from build123d import *

# Parameters (mm, degrees)
SKETCH_1_W          = 117.5
SKETCH_1_H          = 26
EXTRUDE_1_DEPTH     = 1.6
SKETCH_2_R          = 2.2
EXTRUDE_4_DEPTH     = 6.9
SKETCH_3_R          = 1.5
CUT_EXTRUDE_2_DEPTH = 1.6
CUT_EXTRUDE_3_DEPTH = 1.6
SKETCH_5_W          = 20
SKETCH_5_H          = 9
EXTRUDE_5_DEPTH     = 9
SKETCH_6_W          = 18
SKETCH_6_H          = 7
CUT_EXTRUDE_4_DEPTH = 9
FILLET_1_R          = 1.5
CUT_EXTRUDE_5_DEPTH = 1.6
FILLET_2_R          = 1.5


with BuildPart() as part:
    # 草图1 → 凸台-拉伸1 (new body)
    with BuildSketch(Plane.XY):
        Rectangle(SKETCH_1_W, SKETCH_1_H)
    extrude(amount=EXTRUDE_1_DEPTH)

    # 草图2 → 凸台-拉伸4 (add)
    with BuildSketch(Plane.XY.offset(1.6)):
        with Locations((8, 10.25)):
            Circle(SKETCH_2_R)
        with Locations((8, 5.75)):
            Circle(SKETCH_2_R)
        with Locations((24, 10.25)):
            Circle(SKETCH_2_R)
        with Locations((24, 5.75)):
            Circle(SKETCH_2_R)
        with Locations((40, 10.25)):
            Circle(SKETCH_2_R)
        with Locations((40, 5.75)):
            Circle(SKETCH_2_R)
        with Locations((56, 10.25)):
            Circle(SKETCH_2_R)
        with Locations((56, 5.75)):
            Circle(SKETCH_2_R)
        with Locations((-8, 5.75)):
            Circle(SKETCH_2_R)
        with Locations((-8, 10.25)):
            Circle(SKETCH_2_R)
        with Locations((-24, 5.75)):
            Circle(SKETCH_2_R)
        with Locations((-24, 10.25)):
            Circle(SKETCH_2_R)
        with Locations((-40, 5.75)):
            Circle(SKETCH_2_R)
        with Locations((-40, 10.25)):
            Circle(SKETCH_2_R)
        with Locations((-56, 5.75)):
            Circle(SKETCH_2_R)
        with Locations((-56, 10.25)):
            Circle(SKETCH_2_R)
    extrude(amount=EXTRUDE_4_DEPTH)

    # 草图3 → 切除-拉伸2 (cut)
    with BuildSketch(Plane.XY.offset(1.6)):
        with Locations((-15, -9.5)):
            Circle(SKETCH_3_R)
        with Locations((15, -9.5)):
            Circle(SKETCH_3_R)
        with Locations((26, -9.5)):
            Circle(SKETCH_3_R)
        with Locations((-26, -9.5)):
            Circle(SKETCH_3_R)
    extrude(amount=-CUT_EXTRUDE_2_DEPTH, mode=Mode.SUBTRACT)

    # 草图4 → 切除-拉伸3 (cut)
    with BuildSketch(Plane(origin=(0, 0, 0), x_dir=(-1, 0, 0), z_dir=(0, 0, -1))):
        Polygon((-10, -12), (10, -12), (11.75, -13), (0, -13), (-11.75, -13), align=None)
    extrude(amount=-CUT_EXTRUDE_3_DEPTH, mode=Mode.SUBTRACT)

    # 草图5 → 凸台-拉伸5 (add)
    with BuildSketch(Plane(origin=(0, 0, 0), x_dir=(-1, 0, 0), z_dir=(0, 0, -1))):
        with Locations((0, -7.5)):
            Rectangle(SKETCH_5_W, SKETCH_5_H)
    extrude(amount=EXTRUDE_5_DEPTH)

    # 草图6 → 切除-拉伸4 (cut)
    with BuildSketch(Plane(origin=(0, 0, -9), x_dir=(-1, 0, 0), z_dir=(0, 0, -1))):
        with Locations((0, -7.5)):
            Rectangle(SKETCH_6_W, SKETCH_6_H)
    extrude(amount=-CUT_EXTRUDE_4_DEPTH, mode=Mode.SUBTRACT)

    # 圆角1
    fillet_1_edges = [part.edges().sort_by_distance(p)[0] for p in [
        (-58.75, 13, 0.8),
        (58.75, 13, 0.8),
    ]]
    fillet(fillet_1_edges, radius=FILLET_1_R)

    # 草图7 → 切除-拉伸5 (cut)
    with BuildSketch(Plane(origin=(0, 0, 0), x_dir=(-1, 0, 0), z_dir=(0, 0, -1))):
        with BuildLine():
            Line((28, -13), (58.75, -13))
            Line((58.75, -13), (58.75, 1))
            ThreePointArc((58.75, 1), (41.856491631, -2.664704833), (28, -13))
        make_face()
        with BuildLine():
            Line((-58.75, 1), (-58.75, -13))
            Line((-58.75, -13), (-28, -13))
            ThreePointArc((-28, -13), (-41.856491631, -2.664704833), (-58.75, 1))
        make_face()
    extrude(amount=-CUT_EXTRUDE_5_DEPTH, mode=Mode.SUBTRACT)

    # 圆角2
    fillet_2_edges = [part.edges().sort_by_distance(p)[0] for p in [
        (-58.75, 1, 0.8),
        (58.75, 1, 0.8),
    ]]
    fillet(fillet_2_edges, radius=FILLET_2_R)


solid = part.part
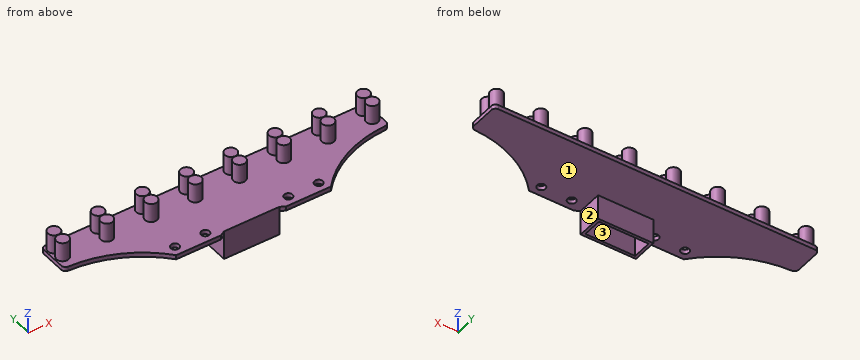
Verification items for the finished model (mm, model axes). Face numbers are marked on the shaded views. Coordinates: 2 decimals unless noted, no trailing zeros. Order: outer loops, then holes, each group sorted by start corner. A loop starts at its lowest first (then second) coordinate and runs counter-clockwise, first axis right, second up. Notation, with made-up numbers: (54.5, -39) -> (92.5, -39) arc R15 ccw to (92.5, -19) -> close; hole circle Ø10 at (-9.5, -16.5). An arc over 180 degrees is marked (long way). Put each result on its own line as item: value. Start each with the question number.
1. Cross-section at B-B, the plane x = 15. Record the boundary of the cut face in (y, z).
2. Cross-section at D-D, the plane y = -9.5. Record the boundary of the cut face in (x, z).
3. Go/stop test with flat-tipped pins: pin 1 Ø1.5 at (x, y) = (-31.5, 3.5) entering from +Z; pin 2 Ø2.5 at (y, z) = (-8, -2.5) entering from +X; pin 3 Ø5 at (x, y) = (-26, -9.5) entering from -Z; pin 4 Ø1.8 at (x, y) = (26, -9.5) entering from +Z. Record where each tip stops, or that it passes through.
4. Material ranges on L1, parallel to Y at x = -8.5, z = -7; L2, parallel to Y at x = -26, z = 0.75; L3, parallel to Z at x = 5.5, y = 9.75, recorded low to high. Write a range as [from, to].
5. Cross-section at A-A, the plane z = 3.75. Count the separate pieces of the cut face and the enclosed holes in it, then the cut area to 3 significant figures.
6. Mould release check, pull along X, two halves, no side actions. Record for the marked faces 1, 2 and 3: released by +X, released by -X, zero draft, split by the parting line, or undercut.
7. Cross-section at C-C, the plane z = -5.75. Record the boundary of the cut face in (x, y).
Computed:
1. outline: (-13, 0) -> (-11, 0) -> (-11, 1.6) -> (-13, 1.6) -> close; (-8, 0) -> (13, 0) -> (13, 1.6) -> (-8, 1.6) -> close
2. outline: (-31.44, 0) -> (-27.5, 0) -> (-27.5, 1.6) -> (-31.44, 1.6) -> close; (-24.5, 0) -> (-16.5, 0) -> (-16.5, 1.6) -> (-24.5, 1.6) -> close; (-13.5, 0) -> (-10, 0) -> (-10, -9) -> (-9, -9) -> (-9, 0) -> (9, 0) -> (9, -9) -> (10, -9) -> (10, 0) -> (13.5, 0) -> (13.5, 1.6) -> (-13.5, 1.6) -> close; (16.5, 0) -> (24.5, 0) -> (24.5, 1.6) -> (16.5, 1.6) -> close; (27.5, 0) -> (31.44, 0) -> (31.44, 1.6) -> (27.5, 1.6) -> close
3. pin 1: z = 1.6
3. pin 2: x = 10
3. pin 3: z = 0
3. pin 4: through
4. L1: [-12, -11], [-4, -3]
4. L2: [-13, -11], [-8, 13]
4. L3: [0, 1.6]
5. separate pieces: 16
5. enclosed holes: 0
5. area: 243 mm2
6. face 1: zero draft
6. face 2: released by +X
6. face 3: undercut
7. outline: (-10, -12) -> (10, -12) -> (10, -3) -> (-10, -3) -> close; hole (-9, -11) -> (9, -11) -> (9, -4) -> (-9, -4) -> close
